from build123d import *

# Parameters (mm, degrees)
BOSS_EXTRU_1_DEPTH                  = 49
ENL_V_MAT_EXTRU_1_REACH             = 107.293
ESQUISSE2_R                         = 2.25
ENL_V_MAT_EXTRU_1_DIRECTION_2_DEPTH = 106.292792514
ENL_V_MAT_EXTRU_2_REACH             = 104.484
ESQUISSE3_R                         = 2.25
ENL_V_START                         = -5
ENL_V_MAT_EXTRU_3_DEPTH             = 5
CONG_1_R                            = 3
ENL_V_START_2                       = -7
ENL_V_MAT_EXTRU_4_DEPTH             = 3.5
BOSS_EXTRU_2_DEPTH                  = 49
CONG_2_R                            = 1.8
CONG_3_R                            = 3
ENL_V_MAT_EXTRU_5_DEPTH             = 102.661483921
ENL_V_MAT_EXTRU_5_DEPTH_BACK        = 102.661483921
ESQUISSE8_W                         = 36
ESQUISSE8_H                         = 16
BOSS_EXTRU_3_START                  = 1.5
ESQUISSE9_R                         = 5.25
ESQUISSE9_R_2                       = 2.25
BOSS_EXTRU_3_DEPTH                  = 1.5
ENL_V_MAT_EXTRU_6_DEPTH             = 3


with BuildPart() as part:
    # Esquisse1 → Boss.-Extru.1 (new body)
    with BuildSketch(Plane.XY):
        Polygon((0, 0), (-28.689142679, 8.771151142), (-30.735744612, 2.07701785), (-24, 0.01769406), (-24, -87.98230594), (-19, -87.98230594), (-19, -1.510959348), (-2.046601933, -6.694133292), align=None)
    extrude(amount=BOSS_EXTRU_1_DEPTH)

    # Esquisse2 → Enlèv. mat.-Extru.1 (cut, up to next)
    with BuildSketch(Plane(origin=(0, 0, 0), x_dir=(0.9563047559630374, -0.2923717047227305, 0), z_dir=(0.2923717047227305, 0.9563047559630374, 0)), mode=Mode.PRIVATE) as enl_v_mat_extru_1_sk1:
        with Locations((-7.5, -9.5)):
            Circle(ESQUISSE2_R)
    enl_v_mat_extru_1_tool1 = extrude(enl_v_mat_extru_1_sk1.sketch, amount=-ENL_V_MAT_EXTRU_1_REACH, mode=Mode.PRIVATE) & part.part
    # Esquisse2 → Enlèv. mat.-Extru.1 (cut, up to next)
    with BuildSketch(Plane(origin=(0, 0, 0), x_dir=(0.9563047559630374, -0.2923717047227305, 0), z_dir=(0.2923717047227305, 0.9563047559630374, 0)), mode=Mode.PRIVATE) as enl_v_mat_extru_1_sk2:
        with Locations((-7.5, -39.5)):
            Circle(ESQUISSE2_R)
    enl_v_mat_extru_1_tool2 = extrude(enl_v_mat_extru_1_sk2.sketch, amount=-ENL_V_MAT_EXTRU_1_REACH, mode=Mode.PRIVATE) & part.part
    add(enl_v_mat_extru_1_tool1.solids().sort_by_distance((-7.172286, 2.192788, 9.5))[0], mode=Mode.SUBTRACT)
    add(enl_v_mat_extru_1_tool2.solids().sort_by_distance((-7.172286, 2.192788, 39.5))[0], mode=Mode.SUBTRACT)

    # Esquisse2 → Enlèv. mat.-Extru.1 direction 2 (cut)
    with BuildSketch(Plane(origin=(0, 0, 0), x_dir=(0.9563047559630374, -0.2923717047227305, 0), z_dir=(0.2923717047227305, 0.9563047559630374, 0))):
        with Locations((-7.5, -9.5)):
            Circle(ESQUISSE2_R)
        with Locations((-7.5, -39.5)):
            Circle(ESQUISSE2_R)
    extrude(amount=ENL_V_MAT_EXTRU_1_DIRECTION_2_DEPTH, mode=Mode.SUBTRACT)

    # Esquisse3 → Enlèv. mat.-Extru.2 (cut, up to next)
    with BuildSketch(Plane(origin=(-19, 0, 0), x_dir=(0, 0, -1), z_dir=(1, 0, 0)), mode=Mode.PRIVATE) as enl_v_mat_extru_2_sk1:
        with Locations((-42.5, -65.98230594)):
            Circle(ESQUISSE3_R)
    enl_v_mat_extru_2_tool1 = extrude(enl_v_mat_extru_2_sk1.sketch, amount=-ENL_V_MAT_EXTRU_2_REACH, mode=Mode.PRIVATE) & part.part
    # Esquisse3 → Enlèv. mat.-Extru.2 (cut, up to next)
    with BuildSketch(Plane(origin=(-19, 0, 0), x_dir=(0, 0, -1), z_dir=(1, 0, 0)), mode=Mode.PRIVATE) as enl_v_mat_extru_2_sk2:
        with Locations(Location((-6.5, -65.98230594, 0), (0, 0, 90))):
            Circle(ESQUISSE3_R)
    enl_v_mat_extru_2_tool2 = extrude(enl_v_mat_extru_2_sk2.sketch, amount=-ENL_V_MAT_EXTRU_2_REACH, mode=Mode.PRIVATE) & part.part
    # Esquisse3 → Enlèv. mat.-Extru.2 (cut, up to next)
    with BuildSketch(Plane(origin=(-19, 0, 0), x_dir=(0, 0, -1), z_dir=(1, 0, 0)), mode=Mode.PRIVATE) as enl_v_mat_extru_2_sk3:
        with Locations((-24.5, -37.98230594)):
            Circle(ESQUISSE3_R)
    enl_v_mat_extru_2_tool3 = extrude(enl_v_mat_extru_2_sk3.sketch, amount=-ENL_V_MAT_EXTRU_2_REACH, mode=Mode.PRIVATE) & part.part
    add(enl_v_mat_extru_2_tool1.solids().sort_by_distance((-19, -65.982306, 42.5))[0], mode=Mode.SUBTRACT)
    add(enl_v_mat_extru_2_tool2.solids().sort_by_distance((-19, -65.982306, 6.5))[0], mode=Mode.SUBTRACT)
    add(enl_v_mat_extru_2_tool3.solids().sort_by_distance((-19, -37.982306, 24.5))[0], mode=Mode.SUBTRACT)

    # Esquisse4 → Enlèv. mat.-Extru.3 (cut)
    with BuildSketch(Plane(origin=(-19, 0, 0), x_dir=(0, 0, -1), z_dir=(1, 0, 0)).offset(ENL_V_START)):
        with BuildLine():
            Line((-24.5, -87.98230594), (-42.5, -72.48230594))
            ThreePointArc((-42.5, -72.48230594), (-47.096194078, -70.578500018), (-49, -65.98230594))
            Line((-49, -65.98230594), (-50, -65.98230594))
            Line((-50, -65.98230594), (-50, -88.98230594))
            Line((-50, -88.98230594), (1, -88.98230594))
            Line((1, -88.98230594), (1, -65.98230594))
            Line((1, -65.98230594), (0, -65.98230594))
            ThreePointArc((0, -65.98230594), (-1.903805922, -70.578500018), (-6.5, -72.48230594))
            Line((-6.5, -72.48230594), (-24.5, -87.98230594))
        make_face()
    extrude(amount=ENL_V_MAT_EXTRU_3_DEPTH, mode=Mode.SUBTRACT)

    # Congé1
    cong_1_edges = [part.edges().sort_by_distance(p)[0] for p in [
        (-21.5, -87.98230594, 24.5),
    ]]
    fillet(cong_1_edges, radius=CONG_1_R)

    # Esquisse5 → Enlèv. mat.-Extru.4 (cut)
    with BuildSketch(Plane(origin=(0, 0, 0), x_dir=(0.9563047559630375, -0.2923717047227304, 0), z_dir=(0.2923717047227304, 0.9563047559630375, 0)).offset(ENL_V_START_2)):
        Polygon((-3.95, -11.549593456), (-3.95, -7.450406544), (-7.5, -5.400813089), (-11.05, -7.450406544), (-11.05, -11.549593456), (-7.5, -13.599186911), align=None)
        Polygon((-7.5, -35.400813089), (-3.95, -37.450406544), (-3.95, -41.549593456), (-7.5, -43.599186911), (-11.05, -41.549593456), (-11.05, -37.450406544), align=None)
    extrude(amount=ENL_V_MAT_EXTRU_4_DEPTH, mode=Mode.SUBTRACT)

    # Esquisse6 → Boss.-Extru.2 (add)
    with BuildSketch(Plane.XY.offset(49)):
        Polygon((-30.735744612, 2.07701785), (-24, -14.98230594), (-24, 0.01769406), align=None)
    extrude(amount=-BOSS_EXTRU_2_DEPTH)

    # Congé2
    cong_2_edges = [part.edges().sort_by_distance(p)[0] for p in [
        (-19, -1.510959348, 24.5),
    ]]
    fillet(cong_2_edges, radius=CONG_2_R)

    # Congé3
    cong_3_edges = [part.edges().sort_by_distance(p)[0] for p in [
        (-29.712443645, 5.424084496, 49),
        (-1.023300967, -3.347066646, 0),
        (-1.023300967, -3.347066646, 49),
        (-29.712443645, 5.424084496, 0),
    ]]
    fillet(cong_3_edges, radius=CONG_3_R)

    # Esquisse8 → Enlèv. mat.-Extru.5 (cut, two sides: drawn at the far end of the back side and taken through both)
    with BuildSketch(Plane(origin=(-19, 0, 0), x_dir=(0, 0, -1), z_dir=(1, 0, 0)).offset(-ENL_V_MAT_EXTRU_5_DEPTH_BACK)):
        with Locations((-24.5, -80.48230594)):
            Rectangle(ESQUISSE8_W, ESQUISSE8_H)
    extrude(amount=ENL_V_MAT_EXTRU_5_DEPTH + ENL_V_MAT_EXTRU_5_DEPTH_BACK, mode=Mode.SUBTRACT)

    # Esquisse9 → Boss.-Extru.3 (add)
    with BuildSketch(Plane(origin=(-19, 0, 0), x_dir=(0, 0, -1), z_dir=(1, 0, 0)).offset(BOSS_EXTRU_3_START)):
        with Locations(Location((-24.5, -37.98230594, 0), (0, 0, 180))):
            Circle(ESQUISSE9_R)
        with Locations(Location((-24.5, -37.98230594, 0), (0, 0, 90))):
            Circle(ESQUISSE9_R_2, mode=Mode.SUBTRACT)
    extrude(amount=-BOSS_EXTRU_3_DEPTH)

    # Esquisse10 → Enlèv. mat.-Extru.6 (cut)
    with BuildSketch(Plane.ZY.offset(24)):
        Polygon((28.05, -40.031899396), (28.05, -35.932712485), (24.5, -33.883119029), (20.95, -35.932712485), (20.95, -40.031899396), (24.5, -42.081492852), align=None)
        Polygon((10.05, -68.031899396), (10.05, -63.932712485), (6.5, -61.883119029), (2.95, -63.932712485), (2.95, -68.031899396), (6.5, -70.081492852), align=None)
        Polygon((46.05, -68.031899396), (46.05, -63.932712485), (42.5, -61.883119029), (38.95, -63.932712485), (38.95, -68.031899396), (42.5, -70.081492852), align=None)
    extrude(amount=-ENL_V_MAT_EXTRU_6_DEPTH, mode=Mode.SUBTRACT)


solid = part.part
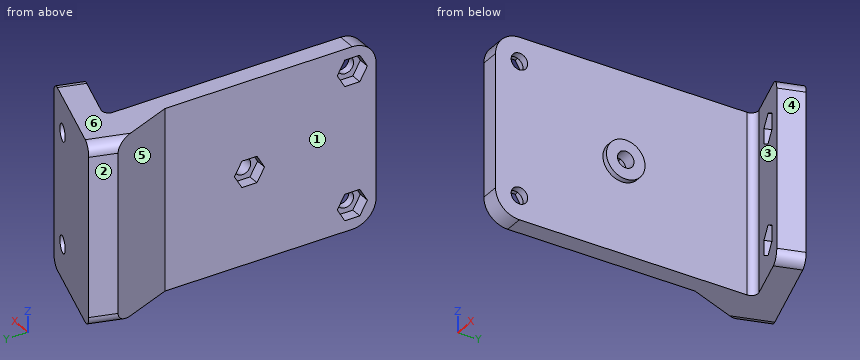
Could you check a few things on this model? Use its own coordinates, in mm. Face numbers are marked on the shaded views. A direction names the side the tool comes from. Coordinates: 2 decimals unless noted, no trailing zeros. Loops run counter-clockwise (first coordinate to the right, second up) from the corner with the lowest first, then second, coordinate; pieces in that order, holes last. Notation, with made-up numbers: (7, 27.25) -> (43, 27.25) arc R14 cw to (43, 33.25) -> close; hole circle Ø7 at (8.25, 49.25). An arc over 180 degrees is marked (long way). Answer in a Markdown table with one row per item.
(1) For the marked faces 1 and 2, which set-ups out of +Z, -Z, +X, -X, +Y, -Y let a thin tool reach every point of the face, with its end or its side?
Results found:
| item | result |
|---|---|
| face 1 | +Z, -Z, -X, -Y |
| face 2 | +Z, -Z, -X, +Y |
(2) Imagine slicing it at B-B (x = -7). Give the number of separate pieces and of enclosed holes in the cut face, plus the area to 3 significant figures.
Results found:
| item | result |
|---|---|
| separate pieces | 3 |
| enclosed holes | 0 |
| area | 283 mm^2 |
(3) Will these pins go through, and if not, where does the flat tip stop? pin 1 Ø5.5 at (y, z) = (-67.5, 6) entering from -X; pin 2 Ø5 at (y, z) = (-65.98, 6.5) entering from +X; pin 3 Ø5 at (y, z) = (-37.98, 24.5) entering from -X.
Results found:
| item | result |
|---|---|
| pin 1 | stops at x = -24 |
| pin 2 | stops at x = -19 |
| pin 3 | stops at x = -21 |
(4) If I drill on probe 1 along Y at (x, z) = (-18.4, 24.5); probe 2 along X at (y, z) = (-53.5, 2); probe 3 along Y at (x, z) = (-20.2, 24.5), over which ranges is the centre line in solid material (lowest first)?
Results found:
| item | result |
|---|---|
| probe 1 | y = -43.23 to -40.23, -35.73 to -32.73, -2.6 to 5.63 |
| probe 2 | x = -24 to -19 |
| probe 3 | y = -72.48 to -40.23, -35.73 to 6.18 |
(5) Imagine slicing it at D-D (x = -13.5). List the corners of the cut face in (y, z) for me.
Results found:
| item | result |
|---|---|
| outline | (-3.19, 0) -> (4.13, 0) -> (4.13, 49) -> (-3.19, 49) -> close |
(6) Thinking about a two-plate mould opening in X: for the marked faces 3, 4, 5 and 6, which applies, released by +X, released by -X, zero draft, split by the parting line, or undercut?
Results found:
| item | result |
|---|---|
| face 3 | undercut |
| face 4 | released by +X |
| face 5 | released by -X |
| face 6 | zero draft |
(7) Imagine slicing it at C-C (y = -49). List the corners of the cut face in (x, z) for me, plus the area to 3 significant figures.
Results found:
| item | result |
|---|---|
| outline | (-24, 0) -> (-19, 0) -> (-19, 49) -> (-24, 49) -> close |
| area | 245 mm^2 |
